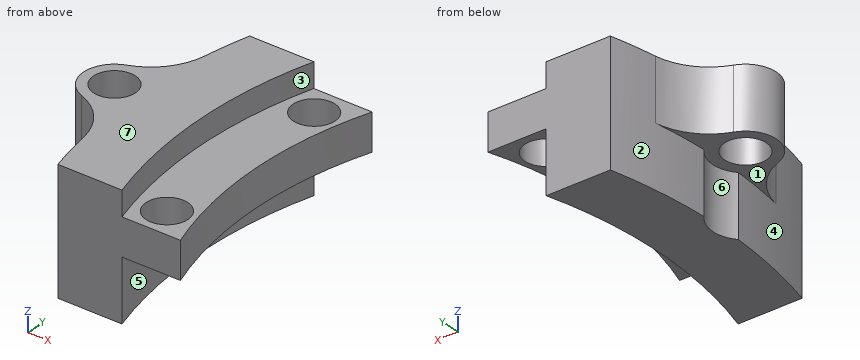
```python
from build123d import *

# Parameters (mm, degrees)
CROQUIS1_R                       = 40.75
CROQUIS1_R_2                     = 35.75
SALIENTE_EXTRUIR1_DEPTH          = 10
CROQUIS2_R                       = 1.7
SALIENTE_EXTRUIR2_DEPTH          = 3
SALIENTE_EXTRUIR3_START          = -5
CROQUIS3_R                       = 1.7
SALIENTE_EXTRUIR3_DEPTH          = 5
CORTAR_EXTRUIR1_DEPTH            = 10
REDONDEO1_R                      = 5
TALADRO_DE_MARGEN_PARA_M51_DEPTH = 5


# Read off the part's stored shape, not the designer's step: Taladro de margen para M51
with BuildPart() as part:
    # Croquis1 → Saliente-Extruir1 (new body)
    with BuildSketch(Plane.XY):
        Circle(CROQUIS1_R)
        Circle(CROQUIS1_R_2, mode=Mode.SUBTRACT)
    extrude(amount=SALIENTE_EXTRUIR1_DEPTH)

    # Croquis2 → Saliente-Extruir2 (add)
    with BuildSketch(Plane(origin=(0, 0, 5), x_dir=(-1, 0, 0), z_dir=(0, 0, -1))):
        with BuildLine():
            Line((34.322915086, -10), (29.606798206, -10))
            ThreePointArc((29.606798206, -10), (31.25, 0), (29.606798206, 10))
            Line((29.606798206, 10), (34.322915086, 10))
            ThreePointArc((34.322915086, 10), (35.75, 0), (34.322915086, -10))
        make_face()
        with Locations((32.492418426, 7.677165354)):
            Circle(CROQUIS2_R, mode=Mode.SUBTRACT)
        with Locations(Location((32.492418426, -7.677165354, 0), (0, 0, 180))):
            Circle(CROQUIS2_R, mode=Mode.SUBTRACT)
    extrude(amount=-SALIENTE_EXTRUIR2_DEPTH)

    # Croquis3 → Saliente-Extruir3 (add)
    with BuildSketch(Plane.XY.offset(10).offset(SALIENTE_EXTRUIR3_START)):
        with BuildLine():
            Line((-40.673240589, -2.5), (-42.673240589, -2.5))
            ThreePointArc((-42.673240589, -2.5), (-45.173240589, 0), (-42.673240589, 2.5))
            Line((-42.673240589, 2.5), (-40.673240589, 2.5))
            ThreePointArc((-40.673240589, 2.5), (-40.75, 0), (-40.673240589, -2.5))
        make_face()
        with Locations((-42.673240589, 0)):
            Circle(CROQUIS3_R, mode=Mode.SUBTRACT)
    extrude(amount=SALIENTE_EXTRUIR3_DEPTH)

    # Croquis4 → Cortar-Extruir1 (cut)
    with BuildSketch(Plane.XY.offset(10)):
        Polygon((-34.322915086, -10), (-63.814245497, -10), (-63.814245497, -44.810382184), (45.541144723, -44.810382184), (45.541144723, 45.96065319), (-49.780136639, 45.96065319), (-49.780136639, 10), (-39.503955498, 10), (-24.875936239, 10), (-24.875936239, -15.19237414), align=None)
    extrude(amount=-CORTAR_EXTRUIR1_DEPTH, mode=Mode.SUBTRACT)

    # Redondeo1
    # the kernel refuses this fillet: 5 mm, written as the material it adds along each edge
    with BuildSketch(Plane(origin=(-40.673240589, -2.5, 5), x_dir=(0.10796118489430687, -0.9941551099080149, 0), z_dir=(0, 0, 1))) as redondeo1_piece_1:
        with BuildLine():
            CenterArc((4.0453205, -4.994529194), REDONDEO1_R, 92.68051287, 61.418565497)
            Line((-0.452433263, -2.810447903), (-0.902208639, -2.592039774))
            ThreePointArc((-0.902208639, -2.592039774), (-0.712999925, -1.934329627), (-0.497077555, 0.053980592))
            Line((-0.497077555, 0.053980592), (0.023383355, 0.499452919))
            ThreePointArc((0.023383355, 0.499452919), (1.905743473, 0.45541293), (3.78810359, 0.499452919))
            Line((3.78810359, 0.499452919), (3.811486945, 0))
        make_face()
    extrude(amount=5)
    with BuildSketch(Plane(origin=(-40.673240589, 2.5, 5), x_dir=(0.1079611848943066, 0.994155109908015, 0), z_dir=(0, 0, 1))) as redondeo1_piece_2:
        with BuildLine():
            CenterArc((4.0453205, 4.994529194), REDONDEO1_R, 205.900921633, 61.418565497)
            Line((-0.452433263, 2.810447903), (-0.902208639, 2.592039774))
            ThreePointArc((-0.902208639, 2.592039774), (-0.712999925, 1.934329627), (-0.497077555, -0.053980592))
            Line((-0.497077555, -0.053980592), (0.023383355, -0.499452919))
            ThreePointArc((0.023383355, -0.499452919), (1.905743473, -0.45541293), (3.78810359, -0.499452919))
            Line((3.78810359, -0.499452919), (3.811486945, 0))
        make_face()
    extrude(amount=5)

    # Taladro de margen para M51 outline → Taladro de margen para M51 (cut)
    with BuildSketch(Plane.XY):
        with BuildLine():
            ThreePointArc((-40.711057028, -1.781105183), (-40.023240589, 0), (-40.711057028, 1.781105183))
            ThreePointArc((-40.711057028, 1.781105183), (-40.75, 0), (-40.711057028, -1.781105183))
        make_face()
    extrude(amount=TALADRO_DE_MARGEN_PARA_M51_DEPTH, mode=Mode.SUBTRACT)


solid = part.part
```
Geometry check sheet. Reference: the model listing, model coordinates, mm. Face numbers are marked on the shaded views. A direction names the side the tool comes from. Round coordinates to 2 decimals unless told otherwise and drop trailing zeros. Loops run counter-clockwise (first coordinate to the right, second up) from the corner with the lowest first, then second, coordinate; pieces in that order, holes last. Notation, with made-up numbers: (51, 11.25) - (90, 11.25) arc R16 ccw to (90, 20.25) - close; hole circle Ø6 at (87.25, 58.5). An arc over 180 degrees is marked (long way). Write item = value, one per line. Start each with the question number.
1. Set-up check for the marked faces 1, 2 and 3: record each of +Z, -Z, +X, -X, +Y, -Y from which the full face is reachable in a straight line by a thin tool's end or side.
2. Section check D-D on z = 6.25. Enter the section's corners in (x, y), then the cut area to 3 significant figures.
3. Section check C-C on x = -42.5. Enter the section's corners in (y, z), then the cut area to 3 significant figures.
4. Section check B-B on z = 9.5. Enter the section's corners in (x, y), then the cut area to 3 significant figures.
5. Mould release check, pull along Y, two halves, no side actions. Record for the marked faces 4, 5, 6 and 7: released by +Y, released by -Y, zero draft, split by the parting line, or undercut.
6. Section check A-A on y = 0. Enter the section's corners in (x, z), then the cut area to 3 significant figures.
7. Thickness scan on line 1 (X direction, y = -8, z = 7.25); line 2 (Z direction, x = -33, y = -3.5); line 3 (X direction, y = 0, z = 2.25). Record the ranges inside material, lowest first.
8. Depth check by flat-ended pin: pin 1 (6 mm diameter, centred on x = -40.5, z = 1.5, fed in from -Y); pin 2 (1.5 mm diameter, centred on x = -42.5, y = -2, fed in from -Z); pin 3 (6 mm diameter, centred on y = 7.5, z = 6, fed in from -X); pin 4 (1.5 mm diameter, centred on y = 6.5, z = 8.5, fed in from -X). Enter the tip coordinate at first touch or a pass-through.
Working result:
q1.face_1 = -Z, -X
q1.face_2 = -Z, -X, +Y
q1.face_3 = +Z, +X
q2.outline = (-43.52, -2.35) arc R5 cw to (-40.26, -6.29) arc R40.75 ccw to (-39.5, -10) - (-29.61, -10) arc R31.25 cw to (-29.61, 10) - (-39.5, 10) arc R40.75 ccw to (-40.26, 6.29) arc R5 cw to (-43.52, 2.35) arc R2.5 ccw to start; hole circle Ø3.4 at (-42.67, 0); hole circle Ø3.4 at (-32.49, -7.68); hole circle Ø3.4 at (-32.49, 7.68)
q2.area = 190 mm^2
q3.outline = (-2.85, 5) - (-1.69, 5) - (-1.69, 10) - (-2.85, 10) - close; (1.69, 5) - (2.85, 5) - (2.85, 10) - (1.69, 10) - close
q3.area = 11.6 mm^2
q4.outline = (-43.52, -2.35) arc R5 cw to (-40.26, -6.29) arc R40.75 ccw to (-39.5, -10) - (-34.32, -10) arc R35.75 cw to (-34.32, 10) - (-39.5, 10) arc R40.75 ccw to (-40.26, 6.29) arc R5 cw to (-43.52, 2.35) arc R2.5 ccw to start; hole circle Ø3.4 at (-42.67, 0)
q4.area = 117 mm^2
q5.face_4 = released by -Y
q5.face_5 = undercut
q5.face_6 = undercut
q5.face_7 = zero draft
q6.outline = (-45.17, 5) - (-44.37, 5) - (-44.37, 10) - (-45.17, 10) - close; (-40.97, 5) - (-40.02, 5) - (-40.02, 0) - (-35.75, 0) - (-35.75, 5) - (-31.25, 5) - (-31.25, 8) - (-35.75, 8) - (-35.75, 10) - (-40.97, 10) - close
q6.area = 65.0 mm^2
q7.line_1 = -39.96 to -34.16, -30.82 to -30.21
q7.line_2 = 5 to 8
q7.line_3 = -40.02 to -35.75
q8.pin_1 = -10
q8.pin_2 = 5
q8.pin_3 = -40.91
q8.pin_4 = -40.38
